```python
from build123d import *

# Parameters (mm, degrees)
SKETCH1_W           = 81.28
SKETCH1_H           = 101.6
BOSS_EXTRUDE1_DEPTH = 2.54
SKETCH2_W           = 27.093333333
SKETCH2_H           = 2.794
CUT_EXTRUDE4_DEPTH  = 66.105308539
SKETCH8_W           = 2.54
SKETCH8_H           = 32.004
CUT_EXTRUDE9_DEPTH  = 66.105308539
SKETCH9_W           = 64.77
SKETCH9_H           = 78.74
CUT_EXTRUDE10_DEPTH = 66.105308539


with BuildPart() as part:
    # Sketch1 → Boss-Extrude1 (new body)
    with BuildSketch(Plane.XY):
        Rectangle(SKETCH1_W, SKETCH1_H)
    extrude(amount=BOSS_EXTRUDE1_DEPTH)

    # Sketch2 → Cut-Extrude4 (cut, through all)
    with BuildSketch(Plane(origin=(0, 0, 0), x_dir=(-1, 0, 0), z_dir=(0, 0, -1))):
        with Locations((27.093333333, -49.403)):
            Rectangle(SKETCH2_W, SKETCH2_H)
        with Locations((-27.093333333, -49.403)):
            Rectangle(SKETCH2_W, SKETCH2_H)
        with Locations((-27.093333333, 49.403)):
            Rectangle(SKETCH2_W, SKETCH2_H)
        with Locations((27.093333333, 49.403)):
            Rectangle(SKETCH2_W, SKETCH2_H)
    extrude(amount=-CUT_EXTRUDE4_DEPTH, mode=Mode.SUBTRACT)

    # Sketch8 → Cut-Extrude9 (cut, through all)
    with BuildSketch(Plane.XY.offset(2.54)):
        with Locations((-39.37, -32.004)):
            Rectangle(SKETCH8_W, SKETCH8_H)
        with Locations((-39.37, 32.004)):
            Rectangle(SKETCH8_W, SKETCH8_H)
        with Locations((39.37, 32.004)):
            Rectangle(SKETCH8_W, SKETCH8_H)
        with Locations((39.37, -32.004)):
            Rectangle(SKETCH8_W, SKETCH8_H)
    extrude(amount=-CUT_EXTRUDE9_DEPTH, mode=Mode.SUBTRACT)

    # Sketch9 → Cut-Extrude10 (cut, through all)
    with BuildSketch(Plane.XY.offset(2.54)):
        Rectangle(SKETCH9_W, SKETCH9_H)
    extrude(amount=-CUT_EXTRUDE10_DEPTH, mode=Mode.SUBTRACT)


solid = part.part
```
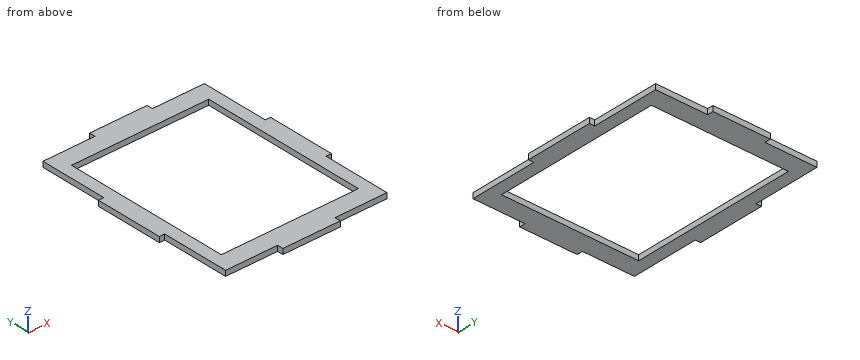
The model under review builds one solid part; all positions refer to its coordinate system, in mm. Round coordinates to 2 decimals unless told otherwise and drop trailing zeros. Loops run counter-clockwise (first coordinate to the right, second up) from the corner with the lowest first, then second, coordinate; pieces in that order, holes last. Notation, with made-up numbers: (-12.5, -9.5) -> (41.5, -9.5) arc R33 cw to (41.5, 29.5) -> close; hole circle Ø5 at (-28.5, 42.25). An arc over 180 degrees is marked (long way). Answer in a Markdown table with one row per item.
1) Consider section C-C, the plane z = 0.5. Write out the cut boundary in (x, y) (3 decimals), plus the area to 3 significant figures.
Taken from the geometry:
| item | result |
|---|---|
| outline | (-40.64, -16.002) -> (-38.1, -16.002) -> (-38.1, -48.006) -> (-13.547, -48.006) -> (-13.547, -50.8) -> (13.547, -50.8) -> (13.547, -48.006) -> (38.1, -48.006) -> (38.1, -16.002) -> (40.64, -16.002) -> (40.64, 16.002) -> (38.1, 16.002) -> (38.1, 48.006) -> (13.547, 48.006) -> (13.547, 50.8) -> (-13.547, 50.8) -> (-13.547, 48.006) -> (-38.1, 48.006) -> (-38.1, 16.002) -> (-40.64, 16.002) -> close; hole (-32.385, -39.37) -> (32.385, -39.37) -> (32.385, 39.37) -> (-32.385, 39.37) -> close |
| area | 2,530 mm² |
2) Consider section A-A, the plane y = -24.5. Write out the cut boundary in (x, z) (3 decimals), plus the area to 3 significant figures.
Taken from the geometry:
| item | result |
|---|---|
| outline | (-38.1, 0) -> (-32.385, 0) -> (-32.385, 2.54) -> (-38.1, 2.54) -> close; (32.385, 0) -> (38.1, 0) -> (38.1, 2.54) -> (32.385, 2.54) -> close |
| area | 29.0 mm² |
3) Wall thickness on line 1 along Y through (x, z) = (15, 1.7); line 2 along X through (y, z) = (24, 0.8) (3 decimals); line 3 along X through (y, z) = (-15, 0.4) (3 decimals): over which ranges is each line inside the solid? List them lowest first.
Taken from the geometry:
| item | result |
|---|---|
| line 1 | y = -48.01 to -39.37, 39.37 to 48.01 |
| line 2 | x = -38.1 to -32.385, 32.385 to 38.1 |
| line 3 | x = -40.64 to -32.385, 32.385 to 40.64 |
4) For pin 1 Ø0.8 at (y, z) = (-36, 1) entering from -X; pin 2 Ø0.8 at (y, z) = (-49, 1) entering from -X; pin 3 Ø0.8 at (x, z) = (-39, 0.5) entering from +Y; pin 4 Ø5 at (x, y) = (25, 35) entering from -Z, all flat-tipped, find the tip position at first contact; note any pin that passes through.
Taken from the geometry:
| item | result |
|---|---|
| pin 1 | stops at x = -38.1 |
| pin 2 | stops at x = -13.55 |
| pin 3 | stops at y = 16 |
| pin 4 | passes through |
5) Consider section B-B, the plane x = 30.5. Write out the cut boundary in (y, z).
Taken from the geometry:
| item | result |
|---|---|
| outline | (-48.01, 0) -> (-39.37, 0) -> (-39.37, 2.54) -> (-48.01, 2.54) -> close; (39.37, 0) -> (48.01, 0) -> (48.01, 2.54) -> (39.37, 2.54) -> close |
